from build123d import *

# Parameters (mm, degrees)
SKETCH2_W           = 167
SKETCH2_H           = 75.5
SKETCH2_R           = 2
BOSS_EXTRUDE1_DEPTH = 5
CUT_EXTRUDE1_DEPTH  = 92.77315784


with BuildPart() as part:
    # Sketch2 → Boss-Extrude1 (new body)
    with BuildSketch(Plane(origin=(0, 0, 0), x_dir=(1, 0, 0), z_dir=(0, 1, 0))):
        Rectangle(SKETCH2_W, SKETCH2_H)
        with Locations(Location((-58.5, 32.75, 0), (0, 0, 270))):
            Circle(SKETCH2_R, mode=Mode.SUBTRACT)
        with Locations(Location((58.5, 32.75, 0), (0, 0, 270))):
            Circle(SKETCH2_R, mode=Mode.SUBTRACT)
        with Locations(Location((-73.5, -4.75, 0), (0, 0, 270))):
            Circle(SKETCH2_R, mode=Mode.SUBTRACT)
        with Locations(Location((73.5, -32.75, 0), (0, 0, 270))):
            Circle(SKETCH2_R, mode=Mode.SUBTRACT)
    extrude(amount=BOSS_EXTRUDE1_DEPTH)

    # Sketch3 → Cut-Extrude1 (cut, through all)
    with BuildSketch(Plane(origin=(0, 5, 0), x_dir=(1, 0, 0), z_dir=(0, 1, 0))):
        with BuildLine():
            ThreePointArc((-29, 7.895643924), (-31.5, 9.5), (-34, 7.895643924))
            Line((-34, 7.895643924), (-34, 5.604356076))
            ThreePointArc((-34, 5.604356076), (-31.5, 4), (-29, 5.604356076))
            Line((-29, 5.604356076), (-29, 7.895643924))
        make_face()
    extrude(amount=-CUT_EXTRUDE1_DEPTH, mode=Mode.SUBTRACT)


solid = part.part
Could you check a few things on this model? Use its own coordinates, in mm. A direction names the side the tool comes from. Round coordinates to 2 decimals unless told otherwise and drop trailing zeros. Write each loop counter-clockwise with the first axis right and the second up, starting at its lowest first coordinate (ties: lowest second). Pieces come first, ordered by that corner, then holes. Notation, with made-up numbers: (34.25, 43) - (41.25, 43) arc R21 cw to (41.25, 79) - close; hole circle Ø11 at (50.5, -27.75). An arc over 180 degrees is marked (long way). Use a Markdown table: item, result.
Q1. Thinking about a two-plate mould opening in Z: for faces 3 (the flat face through (-1, 5, -1)), 4 (the cylindrical face through (-31.5, 2.5, -9.5)), 5 (the flat face through (-1, 2, -37.75)), which applies, released by +Z, released by -Z, zero draft, split by the parting line, or undercut?
Output values:
| item | result |
|---|---|
| face 3 | zero draft |
| face 4 | undercut |
| face 5 | released by -Z |
Q2. I want a section at A-A (z = -32.75). List the corners of the cut face in (x, y) for me.
Output values:
| item | result |
|---|---|
| outline | (-83.5, 0) - (-60.5, 0) - (-60.5, 5) - (-83.5, 5) - close; (-56.5, 0) - (56.5, 0) - (56.5, 5) - (-56.5, 5) - close; (60.5, 0) - (83.5, 0) - (83.5, 5) - (60.5, 5) - close |
Q3. For faces 1 (the cylindrical face through (-31.5, 2.5, -4)), 2 (the flat face through (-1, 0, -1)), which set-ups out of +Z, -Z, +X, -X, +Y, -Y let a thin tool reach every point of the face, with its end or its side?
Output values:
| item | result |
|---|---|
| face 1 | +Y, -Y |
| face 2 | +Z, -Z, +X, -X, -Y |
Q4. Please list where these lines run through material, in increasing order: L1, parallel to X at y = 1.15, z = -32.75; L2, parallel to X at y = 1.95, z = 32.75; L3, parallel to X at y = 2.8, z = 4.75.
Output values:
| item | result |
|---|---|
| L1 | -83.5 to -60.5, -56.5 to 56.5, 60.5 to 83.5 |
| L2 | -83.5 to 71.5, 75.5 to 83.5 |
| L3 | -83.5 to -75.5, -71.5 to 83.5 |
Q5. I want a section at B-B (z = 4.75). List the corners of the cut face in (x, y) for me, plus the area to 3 significant figures.
Output values:
| item | result |
|---|---|
| outline | (-83.5, 0) - (-75.5, 0) - (-75.5, 5) - (-83.5, 5) - close; (-71.5, 0) - (83.5, 0) - (83.5, 5) - (-71.5, 5) - close |
| area | 815 mm2 |
Q6. I want a section at C-C (x = -73.5). List the corners of the cut face in (y, z) for me, plus the area to 4 significant figures.
Output values:
| item | result |
|---|---|
| outline | (0, -37.75) - (5, -37.75) - (5, 2.75) - (0, 2.75) - close; (0, 6.75) - (5, 6.75) - (5, 37.75) - (0, 37.75) - close |
| area | 357.5 mm2 |
